Here's how the part is built. I have some questions about the finished solid (model axes, mm). A direction names the side the tool comes from. Give positions to 0.01 mm unless a question says otherwise; leave off trailing zeros. Write each loop counter-clockwise with the first axis right and the second up, starting at its lowest first coordinate (ties: lowest second). Pieces come first, ordered by that corner, then holes. Notation, with made-up numbers: (57.25, 6.5) -> (62.25, 6.5) arc R6 ccw to (62.25, 11.5) -> close; hole circle Ø11 at (-9.5, 29.5). An arc over 180 degrees is marked (long way). Return JSON: item names as keys, results as strings.
from build123d import *

# Parameters (mm, degrees)
SKETCH1_W           = 284
SKETCH1_H           = 170
BOSS_EXTRUDE1_DEPTH = 65
CUT_EXTRUDE1_DEPTH  = 180
SKETCH3_W           = 30
SKETCH3_H           = 10
BOSS_EXTRUDE2_DEPTH = 90
SKETCH4_W           = 15
SKETCH4_H           = 10
BOSS_EXTRUDE3_DEPTH = 8
CUT_EXTRUDE2_DEPTH  = 10
CUT_EXTRUDE3_DEPTH  = 10
CUT_EXTRUDE4_DEPTH  = 5
SKETCH8_W           = 160
SKETCH8_H           = 40
CUT_EXTRUDE5_DEPTH  = 279
CUT_EXTRUDE6_DEPTH  = 5
SKETCH10_R          = 5
CUT_EXTRUDE7_DEPTH  = 5
FILLET1_R           = 1
FILLET2_R           = 1


with BuildPart() as part:
    # Sketch1 → Boss-Extrude1 (new body)
    with BuildSketch(Plane(origin=(0, 0, 0), x_dir=(1, 0, 0), z_dir=(0, 1, 0))):
        with Locations((142, 85)):
            Rectangle(SKETCH1_W, SKETCH1_H)
    extrude(amount=BOSS_EXTRUDE1_DEPTH)

    # Sketch2 → Cut-Extrude1 (cut)
    with BuildSketch(Plane.ZY):
        Polygon((-140, 52), (-170, 52), (-170, 65), (-150, 65), (-150, 62), (-140, 62), align=None)
        Polygon((-30, 52), (0, 52), (0, 65), (-20, 65), (-20, 62), (-30, 62), align=None)
    extrude(amount=-CUT_EXTRUDE1_DEPTH, mode=Mode.SUBTRACT)

    # Sketch3 → Boss-Extrude2 (add)
    with BuildSketch(Plane.ZY):
        with Locations((-140, 47)):
            Rectangle(SKETCH3_W, SKETCH3_H)
        with Locations((-30, 47)):
            Rectangle(SKETCH3_W, SKETCH3_H)
    extrude(amount=BOSS_EXTRUDE2_DEPTH)

    # Sketch4 → Boss-Extrude3 (add)
    with BuildSketch(Plane(origin=(0, 52, 0), x_dir=(1, 0, 0), z_dir=(0, 1, 0))):
        with Locations((-73, 140)):
            Rectangle(SKETCH4_W, SKETCH4_H)
        with Locations((-73, 30)):
            Rectangle(SKETCH4_W, SKETCH4_H)
    extrude(amount=BOSS_EXTRUDE3_DEPTH)

    # Sketch6 → Cut-Extrude2 (cut)
    with BuildSketch(Plane(origin=(0, 0, -145), x_dir=(-1, 0, 0), z_dir=(0, 0, -1))):
        Polygon((65.5, 60), (80.5, 52), (80.5, 60), align=None)
    extrude(amount=-CUT_EXTRUDE2_DEPTH, mode=Mode.SUBTRACT)

    # Sketch5 → Cut-Extrude3 (cut)
    with BuildSketch(Plane.XY.offset(-25)):
        Polygon((-65.5, 60), (-80.5, 52), (-80.5, 60), align=None)
    extrude(amount=-CUT_EXTRUDE3_DEPTH, mode=Mode.SUBTRACT)

    # Sketch7 → Cut-Extrude4 (cut)
    with BuildSketch(Plane.XZ):
        with BuildLine():
            Line((13.5, -37.5), (13.5, -132.5))
            ThreePointArc((13.5, -132.5), (11, -135), (8.5, -132.5))
            Line((8.5, -132.5), (8.5, -37.5))
            ThreePointArc((8.5, -37.5), (11, -35), (13.5, -37.5))
        make_face()
        with BuildLine():
            Line((58.5, -37.5), (58.5, -132.5))
            ThreePointArc((58.5, -132.5), (56, -135), (53.5, -132.5))
            Line((53.5, -132.5), (53.5, -37.5))
            ThreePointArc((53.5, -37.5), (56, -35), (58.5, -37.5))
        make_face()
        with BuildLine():
            Line((28.5, -37.5), (28.5, -132.5))
            ThreePointArc((28.5, -132.5), (26, -135), (23.5, -132.5))
            Line((23.5, -132.5), (23.5, -37.5))
            ThreePointArc((23.5, -37.5), (26, -35), (28.5, -37.5))
        make_face()
        with BuildLine():
            Line((43.5, -37.5), (43.5, -132.5))
            ThreePointArc((43.5, -132.5), (41, -135), (38.5, -132.5))
            Line((38.5, -132.5), (38.5, -37.5))
            ThreePointArc((38.5, -37.5), (41, -35), (43.5, -37.5))
        make_face()
    extrude(amount=-CUT_EXTRUDE4_DEPTH, mode=Mode.SUBTRACT)

    # Sketch8 → Cut-Extrude5 (cut)
    with BuildSketch(Plane(origin=(284, 0, 0), x_dir=(0, 0, -1), z_dir=(1, 0, 0))):
        with Locations((85, 25)):
            Rectangle(SKETCH8_W, SKETCH8_H)
    extrude(amount=-CUT_EXTRUDE5_DEPTH, mode=Mode.SUBTRACT)

    # Sketch9 → Cut-Extrude6 (cut)
    with BuildSketch(Plane.XY):
        Polygon((219.15, 25.8), (229.05, 25.8), (229.05, 8.15), (226.8, 5), (221.4, 5), (219.15, 8.15), align=None)
        Polygon((164.25, 25.8), (174.15, 25.8), (174.15, 8.15), (171.9, 5), (166.5, 5), (164.25, 8.15), align=None)
    extrude(amount=-CUT_EXTRUDE6_DEPTH, mode=Mode.SUBTRACT)

    # Sketch10 → Cut-Extrude7 (cut)
    with BuildSketch(Plane.ZY):
        with Locations((-129.202249563, 20)):
            Circle(SKETCH10_R)
        with Locations((-114.202249563, 20)):
            Circle(SKETCH10_R)
        with Locations((-99.202249563, 20)):
            Circle(SKETCH10_R)
        with Locations((-43.390057257, 20)):
            Circle(SKETCH10_R)
        with Locations((-58.390057257, 20)):
            Circle(SKETCH10_R)
        with Locations((-73.390057257, 20)):
            Circle(SKETCH10_R)
    extrude(amount=-CUT_EXTRUDE7_DEPTH, mode=Mode.SUBTRACT)

    # Fillet1
    fillet1_edges = [part.edges().sort_by_distance(p)[0] for p in [
        (0, 65, -85),
        (0, 63.5, -150),
        (0, 62, -145),
        (0, 62, -25),
        (0, 63.5, -20),
    ]]
    fillet(fillet1_edges, radius=FILLET1_R)

    # Fillet2
    fillet2_edges = [part.edges().sort_by_distance(p)[0] for p in [
        (284, 65, -85),
        (142, 0, -170),
        (284, 0, -85),
        (142, 0, 0),
        (0, 0, -85),
        (284, 32.5, -170),
        (284, 32.5, 0),
    ]]
    fillet(fillet2_edges, radius=FILLET2_R)


solid = part.part
1. For pin 1 Ø9 at (x, y) = (-71.5, 56) entering from -Z; pin 2 Ø12 at (y, z) = (20.5, -119.5) entering from +X; pin 3 Ø3.5 at (x, y) = (102.5, 64) entering from +Z, each with a flat end and sliding along its axis, tell me the tip position at first contact or that it passes through.
Taken from the geometry:
{"pin 1": "stops at z = -155", "pin 2": "stops at x = 5", "pin 3": "stops at z = -20"}
2. Which directions (+Z, -Z, +X, -X, +Y, -Y) give clear straight access to the entire face, cutting with the end or side of a thin tool? Please do faces 4 (the face through (89, 62, -25)), 5 (the face through (180, 59, -15)), 6 (the face through (-44, 47, -15)), 7 (the face through (-44, 47, -125)).
Taken from the geometry:
{"face 4": "+Z, -X", "face 5": "+Z", "face 6": "+Z, -X, +Y, -Y", "face 7": "-X, +Y, -Y"}
3. If I drill on line 1 (Y direction, x = 94, z = -97.5); line 2 (Y direction, x = 157, z = -153); line 3 (Y direction, x = 77, z = -147), over which ranges is the centre line in solid material (lowest first)? Write a range as [from, to].
Taken from the geometry:
{"line 1": "y = [0, 5], [45, 65]", "line 2": "y = [0, 5], [45, 52]", "line 3": "y = [0, 5], [45, 52], [62, 65]"}
4. Suppose I cut it at A-A, the plane x = -22. List the corners of the cut face in (y, z) for me.
Taken from the geometry:
{"outline": "(42, -155) -> (52, -155) -> (52, -125) -> (42, -125) -> close; (42, -45) -> (52, -45) -> (52, -15) -> (42, -15) -> close"}
5. If we mould it in two halves opening along X, with no side actions, what happens to faces 1 (the face through (-65.5, 56, -30)), 2 (the face through (-90, 47, -140)), 3 (the face through (-44, 42, -30))? For each: released by +X, released by -X, zero draft, split by the parting line, or undercut.
Taken from the geometry:
{"face 1": "undercut", "face 2": "released by -X", "face 3": "zero draft"}
6. Suppose I cut it at B-B, the plane x = 90.5. List the corners of the cut face in (y, z) for me.
Taken from the geometry:
{"outline": "(0, -169) arc R1 ccw to (1, -170) -> (52, -170) -> (52, -140) -> (62, -140) -> (62, -150) -> (65, -150) -> (65, -20) -> (62, -20) -> (62, -30) -> (52, -30) -> (52, 0) -> (1, 0) arc R1 ccw to (0, -1) -> close; hole (5, -165) -> (45, -165) -> (45, -5) -> (5, -5) -> close"}
7. Suppose I cut it at C-C, the plane y = 20. Count the separate pieces of the cut face and the enclosed holes in it, and give its area (3 significant figures).
Taken from the geometry:
{"separate pieces": "9", "enclosed holes": "0", "area": "3,240 mm²"}
